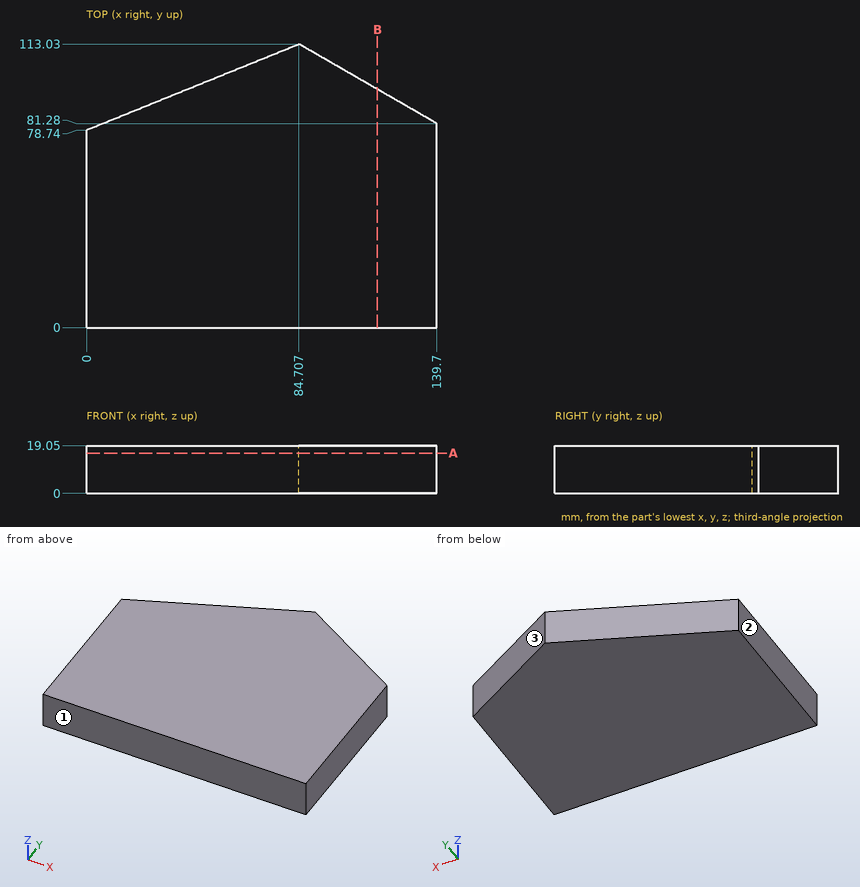
Geometry check sheet. Reference: drawing and pictorial views, mm from the part's lowest x, y, z. Coordinates: 2 decimals unless noted, no trailing zeros. Order: outer loops, then holes, each group sorted by start corner. A loop starts at its lowest first (then second) coordinate and runs counter-clockwise, first axis right, second up.
1. Sectioned sample at B-B, the plane x = 116. Record the cut outline in (y, z).
Results found:
outline: (0, 0) - (94.96, 0) - (94.96, 19.05) - (0, 19.05) - close
2. Scan lines: line 1 (X direction, y = 99.5, z = 17) (1 decimal); line 2 (Y direction, x = 52.5, z = 3); line 3 (Y direction, x = 75, z = 5). Record each from-to range of solid material in increasing order.
Results found:
line 1: x = 51.3 to 108.1
line 2: y = 0 to 99.99
line 3: y = 0 to 109.1
3. Release check for a two-part mould opening along Y. For the marked faces 1, 2 and 3 record: +Y half, -Y half, draft (parallel to the pull), parting line (faces both ways), or undercut.
Results found:
face 1: -Y half
face 2: draft
face 3: +Y half
4. Sectioned sample at A-A, the plane z = 16. Record the cut outline in (x, y), and give its area (3 significant figures).
Results found:
outline: (0, 0) - (139.7, 0) - (139.7, 81.28) - (84.71, 113.03) - (0, 78.74) - close
area: 13,500 mm2
5. Go/stop test with flat-tipped pins: pin 1 Ø5 at (x, z) = (93.5, 9) entering from +Y; pin 2 Ø5 at (x, z) = (49.5, 16.5) entering from +Y; pin 3 Ø2 at (x, z) = (79, 9) entering from +Y (1 decimal). Record where each tip stops, or that it passes through.
Results found:
pin 1: stops at y = 109.4
pin 2: stops at y = 99.79
pin 3: stops at y = 111.1
